Source: three-view drawing plus pictorial views. Frame: mm from the lowest corner of the part. A direction names the side the tool comes from. Give positions to 0.01 mm unless a question says otherwise; leave off trailing zeros. Order: outer loops, then holes, each group sorted by start corner. A loop starts at its lowest first (then second) coordinate and runs counter-clockwise, first axis right, second up. Notation, with made-up numbers: (-14.75, 57) -> (20.25, 57) arc R15 cw to (20.25, 63) -> close; hole circle Ø9 at (61.25, 17). An arc over 180 degrees is marked (long way). Answer in a Markdown table with one row per item. Add a question column.
Q1. Cut plane B-B on x = 692. Return the cut outline in (y, z).
Q2. Cut plane A-A on z = 22. Return the cut outline in (x, y).
Q3. Cut plane C-C on y = 13. Return the cut outline in (x, z), and give its area (3 significant figures).
Q4. Set-up query: the marked faces 1, 2 and 3. Return all of +Z, -Z, +X, -X, +Y, -Y with unobstructed straight access to the full face (end or side cutting, diameter ignored); none if empty.
Q5. Contact query for flat-ended pins moving along their axis: P1, Ø5, axis at x = 790.5, z = 128, coming from the -Y side; P2, Ø3, axis at y = 71, z = 149, coming from the -X side; P3, Ø6, axis at y = 96, z = 43.5, coming from the +X side (1 decimal). Output: stop coordinate, or through.
Q6. Line query: line 1 along X through (y, z) = (120, 142.5); line 2 along Y through (x, z) = (240, 107); line 3 along Y through (x, z) = (880, 130). Output: solid intervals per line, ascending. Write a range as from..to.
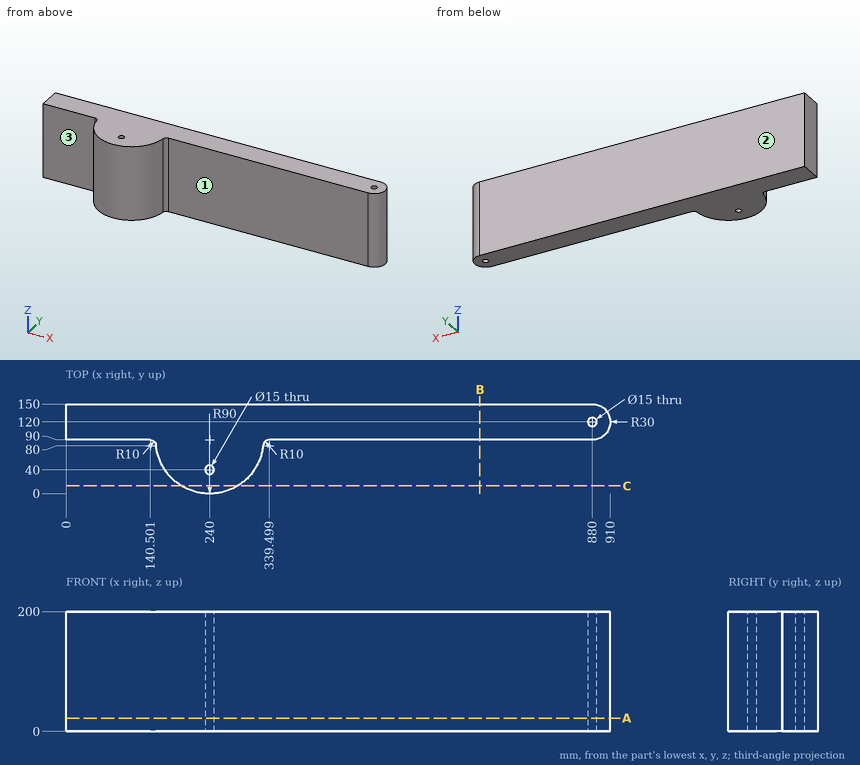
Completed:
| question | item | result |
|---|---|---|
| 1 | outline | (90, 0) -> (150, 0) -> (150, 200) -> (90, 200) -> close |
| 2 | outline | (0, 90) -> (140.5, 90) arc R10 cw to (150.45, 81) arc R90 ccw to (329.55, 81) arc R10 cw to (339.5, 90) -> (880, 90) arc R30 ccw to (880, 150) -> (0, 150) -> close; hole circle Ø15 at (240, 40); hole circle Ø15 at (880, 120) |
| 3 | outline | (193.41, 0) -> (286.59, 0) -> (286.59, 200) -> (193.41, 200) -> close |
| 3 | area | 18,600 mm² |
| 4 | face 1 | +Z, -Z, +X, -Y |
| 4 | face 2 | +Z, -Z, +X, -X, +Y |
| 4 | face 3 | +Z, -Z, -X, -Y |
| 5 | P1 | stops at y = 90 |
| 5 | P2 | stops at x = 151.72 |
| 5 | P3 | stops at x = 901.4 |
| 6 | line 1 | x = 0..872.5, 887.5..910 |
| 6 | line 2 | y = 0..32.5, 47.5..150 |
| 6 | line 3 | y = 90..112.5, 127.5..150 |
